Read the model definition and answer for the solid it produces. Units are mm, in the model's axes. Round coordinates to 2 decimals unless told otherwise and drop trailing zeros. Loops run counter-clockwise (first coordinate to the right, second up) from the corner with the lowest first, then second, coordinate; pieces in that order, holes last. Notation, with made-up numbers: M -26.75,59.5 L 17.25,59.5 A22 ccw 17.25,93.5 Z; hole C -3,-22.5 d5. An arc over 180 degrees is marked long. Write each question's results on one line, items separated by ' | '.
from build123d import *

# Parameters (mm, degrees)
F0_R     = 48
F1_DEPTH = 3
F2_R     = 48
F2_R_2   = 45
F3_DEPTH = 4
F4_SIZE  = 0.8
F6_DEPTH = 1.5


with BuildPart() as f1:
    # F0 (on Top) → F1 (new body)
    with BuildSketch(Plane.XY):
        Circle(F0_R)
    extrude(amount=F1_DEPTH)

    # F2 (on Top) → F3 (join)
    with BuildSketch(Plane.XY):
        Circle(F2_R)
        Circle(F2_R_2, mode=Mode.SUBTRACT)
    extrude(amount=F3_DEPTH)

    # F4
    f4_edges = [f1.edges().sort_by_distance(p)[0] for p in [
        (-48, 0, 4),
        (-45, 0, 4),
    ]]
    chamfer(f4_edges, length=F4_SIZE)

    # F5 (on face) → F6 (cut)
    with BuildSketch(Plane.XY.offset(3)):
        with BuildLine():
            ThreePointArc((0, -25), (-12.5, -12.5), (0, 0))
            ThreePointArc((0, 0), (12.5, 12.5), (0, 25))
            ThreePointArc((0, 25), (-25, 0), (0, -25))
        make_face()
    extrude(amount=-F6_DEPTH, mode=Mode.SUBTRACT)


solid = f1.part
Item 1: Flat-ended cylindrical pins translate along their axes: pin 1 (1.5 mm diameter, centred on x = 22.5, y = 34.5, fed in from +Z); pin 2 (1.5 mm diameter, centred on y = -9, z = 2.5, fed in from -X); pin 3 (1.5 mm diameter, centred on x = -33.5, y = -16, fed in from -Z); pin 4 (2 mm diameter, centred on y = -25.5, z = 2, fed in from +X). Find the tip coordinate at first contact, or state that the pin passes through.
Outcome:
pin 1: stops at z = 3 | pin 2: stops at x = -47.29 | pin 3: stops at z = 0 | pin 4: stops at x = 41.28
Item 2: Straight lines are drawn through the part: line 1 (Y direction, x = 0, z = 3.1); line 2 (Z direction, x = 2.5, y = -32); line 3 (X direction, y = -10.5, z = 1.75). For each, find the intervals that lie inside material, in ascending order.
Outcome:
line 1: y = -48 to -45, 45 to 48 | line 2: z = 0 to 3 | line 3: x = -46.84 to -22.69, -12.34 to 46.84
Item 3: The mould has two halves that part along Y. Classify faces 1 (the face through (-1, 1, 0)), 2 (the face through (9, 1, 3)), 3 (the face through (-7, 6, 1.5)), 4 (the face through (-47.954, 2.11, 1.578)): pulls with the +Y half, pulls with the -Y half, needs draft (parallel to the pull), parting line crosses it, or undercut.
Outcome:
face 1: needs draft | face 2: undercut | face 3: undercut | face 4: parting line crosses it
Item 4: The part is cut by section A-A (z = 0.6). Determine the outline of the cut face in (x, y), plus the area to 3 significant figures.
Outcome:
outline: C 0,0 d96 | area: 7,240 mm2
